Build history of the part. All positions in model axes, mm. A direction names the side the tool comes from. Give positions to 0.01 mm unless a question says otherwise; leave off trailing zeros. Order: outer loops, then holes, each group sorted by start corner. A loop starts at its lowest first (then second) coordinate and runs counter-clockwise, first axis right, second up. Notation, with made-up numbers: (30, 28) - (85, 28) arc R26 ccw to (85, 56) - close; hole circle Ø6 at (60, 32). An arc over 180 degrees is marked (long way). Answer in a Markdown table with one row per item.
```python
from build123d import *

# Parameters (mm, degrees)
F0_W     = 84
F0_H     = 9
F0_R     = 1.5
F0_W_2   = 72
F0_H_2   = 3
F0_H_3   = 4
F1_DEPTH = 2
F2_W     = 84
F2_H     = 2
F3_DEPTH = 9
F4_R     = 1.5
F5_DEPTH = 25


with BuildPart() as f1:
    # F0 (on Front) → F1 (new body)
    with BuildSketch(Plane.XZ):
        Rectangle(F0_W, F0_H)
        with Locations((-37.5, 0)):
            Circle(F0_R, mode=Mode.SUBTRACT)
        with Locations((3, 0)):
            Rectangle(F0_W_2, F0_H_2, mode=Mode.SUBTRACT)
        with Locations((0, 6.5)):
            Rectangle(F0_W, F0_H_3)
    extrude(amount=F1_DEPTH)

    # F2 (on face) → F3 (join)
    with BuildSketch(Plane.XZ.offset(2)):
        with Locations((0, 7.5)):
            Rectangle(F2_W, F2_H)
    extrude(amount=F3_DEPTH)

    # F4 (on face) → F5 (cut)
    with BuildSketch(Plane.XY.offset(8.5)):
        with Locations((0, -6.5)):
            Circle(F4_R)
        with Locations((33, -6.5)):
            Circle(F4_R)
        with Locations((-33, -6.5)):
            Circle(F4_R)
    extrude(amount=-F5_DEPTH, mode=Mode.SUBTRACT)


solid = f1.part
```
1. Cut at D-D on x = 20. Write the cut outline in (y, z).
Check result:
| item | result |
|---|---|
| outline | (-11, 6.5) - (-2, 6.5) - (-2, 1.5) - (0, 1.5) - (0, 8.5) - (-11, 8.5) - close; (-2, -4.5) - (0, -4.5) - (0, -1.5) - (-2, -1.5) - close |
2. Cut at B-B on z = 0. Write the cut outline in (x, y).
Check result:
| item | result |
|---|---|
| outline | (-42, -2) - (-39, -2) - (-39, 0) - (-42, 0) - close; (-36, -2) - (-33, -2) - (-33, 0) - (-36, 0) - close; (39, -2) - (42, -2) - (42, 0) - (39, 0) - close |
3. Probe line 1 (Y direction, x = 33, z = 7.25); line 2 (Y direction, x = 19, z = 4); line 3 (Z direction, x = -37.5, y = -1.45). List the from-to ranges inside material, lowest first.
Check result:
| item | result |
|---|---|
| line 1 | y = -11 to -8, -5 to 0 |
| line 2 | y = -2 to 0 |
| line 3 | z = -4.5 to -1.5, 1.5 to 8.5 |
4. Which spindle directions (+Z, -Z, +X, -X, +Y, -Y) get a long thin tool onto all of the face, cutting with end or side? Do faces 5 (the face through (-1, -8, 6.5)), 6 (the face through (39, -1, 0)), 7 (the face through (-1, -1, -4.5)). Say none if no direction does.
Check result:
| item | result |
|---|---|
| face 5 | -Z, +X, -X, -Y |
| face 6 | +Y, -Y |
| face 7 | -Z, +X, -X, +Y, -Y |
5. Two-plate mould, pull along Y, no slides. Class faces 1 (the face through (31.5, -6.43, 7.51)), 2 (the face through (0, -8, 8)), 3 (the face through (-42, -1, 4)), 4 (the face through (-1, -2, 2)): +Y half, -Y half, draft (parallel to the pull), parting line (faces both ways), or undercut.
Check result:
| item | result |
|---|---|
| face 1 | undercut |
| face 2 | undercut |
| face 3 | draft |
| face 4 | -Y half |
6. Cut at C-C on y = -6.5. Write the cut outline in (x, z).
Check result:
| item | result |
|---|---|
| outline | (-42, 6.5) - (-34.5, 6.5) - (-34.5, 8.5) - (-42, 8.5) - close; (-31.5, 6.5) - (-1.5, 6.5) - (-1.5, 8.5) - (-31.5, 8.5) - close; (1.5, 6.5) - (31.5, 6.5) - (31.5, 8.5) - (1.5, 8.5) - close; (34.5, 6.5) - (42, 6.5) - (42, 8.5) - (34.5, 8.5) - close |
7. Cut at A-A on x = 0. Write the cut outline in (y, z), and give its area (3 significant figures).
Check result:
| item | result |
|---|---|
| outline | (-11, 6.5) - (-8, 6.5) - (-8, 8.5) - (-11, 8.5) - close; (-5, 6.5) - (-2, 6.5) - (-2, 1.5) - (0, 1.5) - (0, 8.5) - (-5, 8.5) - close; (-2, -4.5) - (0, -4.5) - (0, -1.5) - (-2, -1.5) - close |
| area | 32.0 mm² |
8. Drop flat-ended pins along their axis: P1, Ø1.5, axis at x = 0, y = -9, coming from the -Z side; P2, Ø5, axis at x = 33, y = -6.5, coming from the +Z side. Give the stop position or say it passes through.
Check result:
| item | result |
|---|---|
| P1 | stops at z = 6.5 |
| P2 | stops at z = 8.5 |
